CAD build for the part. Positions are in the model's coordinates, mm. Face numbers are marked on the shaded views. A direction names the side the tool comes from. Coordinates: 2 decimals unless noted, no trailing zeros. Loops run counter-clockwise (first coordinate to the right, second up) from the corner with the lowest first, then second, coordinate; pieces in that order, holes last. Notation, with made-up numbers: (-38.75, 78.25) -> (8.25, 78.25) arc R34 ccw to (8.25, 110.25) -> close; hole circle Ø4 at (-25.75, -32). An arc over 180 degrees is marked (long way). Answer as CSV lines item,"result". Start each with the question number.
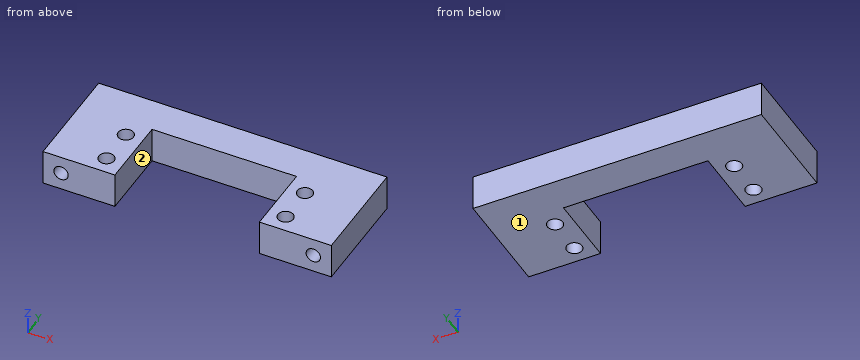
```python
from build123d import *

# Parameters (mm, degrees)
BOSS_EXTRUDE1_DEPTH = 10
SKETCH2_R           = 2
CUT_EXTRUDE1_DEPTH  = 15
SKETCH3_R           = 2.125
CUT_EXTRUDE2_DEPTH  = 87.02325267


with BuildPart() as part:
    # Sketch1 → Boss-Extrude1 (new body)
    with BuildSketch(Plane.XY):
        Polygon((0, 0), (19.95, 0), (19.95, 20), (60.05, 20), (60.05, 0), (80, 0), (80, 30), (0, 30), align=None)
    extrude(amount=BOSS_EXTRUDE1_DEPTH)

    # Sketch2 → Cut-Extrude1 (cut)
    with BuildSketch(Plane.XZ):
        with Locations(Location((5, 5, 0), (0, 0, 270))):
            Circle(SKETCH2_R)
        with Locations(Location((75, 5, 0), (0, 0, 270))):
            Circle(SKETCH2_R)
    extrude(amount=-CUT_EXTRUDE1_DEPTH, mode=Mode.SUBTRACT)

    # Sketch3 → Cut-Extrude2 (cut, through all)
    with BuildSketch(Plane.XY.offset(10)):
        with Locations((15.15, 4.8)):
            Circle(SKETCH3_R)
        with Locations((15.15, 15.2)):
            Circle(SKETCH3_R)
        with Locations(Location((64.85, 15.2, 0), (0, 0, 180))):
            Circle(SKETCH3_R)
        with Locations(Location((64.85, 4.8, 0), (0, 0, 180))):
            Circle(SKETCH3_R)
    extrude(amount=-CUT_EXTRUDE2_DEPTH, mode=Mode.SUBTRACT)


solid = part.part
```
Q1. Saw through at A-A (y = 4.8). List the corners of the cut face in (x, z) (3 decimals), and give its area (3 significant figures).
Q2. Saw through at D-D (x = 75). List the corners of the cut face in (y, z).
Q3. Probe probe 1 along Y at (x, z) = (15.15, 5.5) (3 decimals); probe 2 along X at (y, z) = (9.5, 5); probe 3 along X at (y, z) = (13.25, 8.25). List the from-to ranges inside material, lowest first. Write a range as from..to.
Q4. Saw through at C-C (z = 8). List the corners of the cut face in (x, y) (3 decimals), and give its area (3 significant figures).
Q5. Pin check, flat tips, straight feed: pin 1 Ø3 at (x, z) = (49.5, 6) entering from -Y; pin 2 Ø6 at (y, z) = (24, 9) entering from -X. Stop position of each tip, or through.
Q6. Which spindle directions (+Z, -Z, +X, -X, +Y, -Y) get a long thin tool onto all of the face, cutting with end or side? Do the marked faces 1 and 2. Say none if no direction does.
Q7. Saw through at B-B (x = 64.85). List the corners of the cut face in (y, z) (3 decimals).
Ans:
1,outline,"(0, 0) -> (13.025, 0) -> (13.025, 10) -> (0, 10) -> close; (17.275, 0) -> (19.95, 0) -> (19.95, 10) -> (17.275, 10) -> close; (60.05, 0) -> (62.725, 0) -> (62.725, 10) -> (60.05, 10) -> close; (66.975, 0) -> (80, 0) -> (80, 10) -> (66.975, 10) -> close; hole circle Ø4 at (5, 5); hole circle Ø4 at (75, 5)"
1,area,"289 mm²"
2,outline,"(0, 0) -> (30, 0) -> (30, 10) -> (0, 10) -> (0, 7) -> (15, 7) -> (15, 3) -> (0, 3) -> close"
3,probe 1,"y = 0..2.675, 6.925..13.075, 17.325..30"
3,probe 2,"x = 0..3, 7..19.95, 60.05..73, 77..80"
3,probe 3,"x = 0..14.31, 15.99..19.95, 60.05..64.01, 65.69..80"
4,outline,"(0, 0) -> (19.95, 0) -> (19.95, 20) -> (60.05, 20) -> (60.05, 0) -> (80, 0) -> (80, 30) -> (0, 30) -> close; hole circle Ø4.25 at (15.15, 4.8); hole circle Ø4.25 at (15.15, 15.2); hole circle Ø4.25 at (64.85, 4.8); hole circle Ø4.25 at (64.85, 15.2)"
4,area,"1,540 mm²"
5,pin 1,"stops at y = 20"
5,pin 2,"stops at x = 0"
6,face 1,"-Z, +X, -X, +Y, -Y"
6,face 2,"+Z, -Z, -Y"
7,outline,"(0, 0) -> (2.675, 0) -> (2.675, 10) -> (0, 10) -> close; (6.925, 0) -> (13.075, 0) -> (13.075, 10) -> (6.925, 10) -> close; (17.325, 0) -> (30, 0) -> (30, 10) -> (17.325, 10) -> close"
